from build123d import *

# Parameters (mm, degrees)
SM_BASE_FLANGE_2_DEPTH = 20
HOLE_WIZARD_M3_1_D     = 3.2
SKETCH_24_R            = 3.6
CUT_EXTRUDE_2_DEPTH    = 67.332495807
HOLE_WIZARD_M4_1_D     = 4.3
HOLE_WIZARD_M2_5_1_D   = 2.7


# Sheet-metal steps are written as plain solids
with BuildPart() as part:
    # 草圖16 → 基材-凸緣2 (new, symmetric)
    with BuildSketch(Plane.XY):
        with BuildLine():
            Line((36, 0), (1, 0))
            ThreePointArc((1, 0), (0.292893219, 0.292893219), (0, 1))
            Line((0, 1), (0, 48))
            Line((0, 48), (-4, 48))
            Line((-4, 48), (-4, 1))
            ThreePointArc((-4, 1), (-2.535533906, -2.535533906), (1, -4))
            Line((1, -4), (36, -4))
            Line((36, -4), (36, 0))
        make_face()
    extrude(amount=SM_BASE_FLANGE_2_DEPTH, both=True)

    # M3 餘隙孔1 (through all)
    with Locations(Plane(origin=(0, 0, 0), x_dir=(-1, 0, 0), z_dir=(0, 1, 0))):
        with Locations((-27, 17.5), (-11, 2.5), (-11, 17.5), (-27, 2.5)):
            Hole(HOLE_WIZARD_M3_1_D / 2)

    # 草圖24 → 除料-伸長2 (cut, through all)
    with BuildSketch(Plane.XZ.offset(4)):
        with Locations(Location((19, -10, 0), (0, 0, 270))):
            Circle(SKETCH_24_R)
    extrude(amount=-CUT_EXTRUDE_2_DEPTH, mode=Mode.SUBTRACT)

    # M4 餘隙孔1 (through all)
    with Locations(Plane(origin=(0, 0, 0), x_dir=(0, 0, 1), z_dir=(1, 0, 0))):
        with Locations((0, -44), (15, -44), (15, -24), (0, -24)):
            Hole(HOLE_WIZARD_M4_1_D / 2)

    # M2.5 餘隙孔1 (through all)
    with Locations(Plane(origin=(0, -4, 0), x_dir=(-1, 0, 0), z_dir=(0, -1, 0))):
        with Locations((-11.5, 10), (-26.5, 10)):
            Hole(HOLE_WIZARD_M2_5_1_D / 2)


solid = part.part
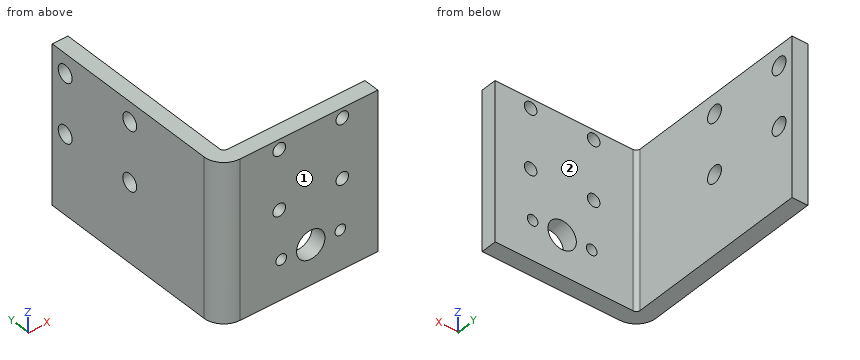
Build history of the part. All positions in model axes, mm. Face numbers are marked on the shaded views. A direction names the side the tool comes from. Round coordinates to 2 decimals unless told otherwise and drop trailing zeros. Loops run counter-clockwise (first coordinate to the right, second up) from the corner with the lowest first, then second, coordinate; pieces in that order, holes last. Notation, with made-up numbers: (74, -10.75) -> (121, -10.75) arc R17 ccw to (121, 13.25) -> close; hole circle Ø7 at (0, 57). An arc over 180 degrees is marked (long way). Answer in a Markdown table with one row per item.
Item 1: Which spindle directions (+Z, -Z, +X, -X, +Y, -Y) get a long thin tool onto all of the face, cutting with end or side? Do the marked faces 1 and 2. Say none if no direction does.
Answers below:
| item | result |
|---|---|
| face 1 | +Z, -Z, +X, -X, -Y |
| face 2 | +Z, -Z, +X, +Y |
Item 2: Saw through at B-B (x = 27). Write the cut outline in (y, z), and give its area (3 significant figures).
Answers below:
| item | result |
|---|---|
| outline | (-4, -20) -> (0, -20) -> (0, -11.25) -> (-4, -11.25) -> close; (-4, -8.75) -> (0, -8.75) -> (0, 0.9) -> (-4, 0.9) -> close; (-4, 4.1) -> (0, 4.1) -> (0, 15.9) -> (-4, 15.9) -> close; (-4, 19.1) -> (0, 19.1) -> (0, 20) -> (-4, 20) -> close |
| area | 124 mm² |
Item 3: Saw through at D-D (z = -10). Write the cut outline in (x, y), and give its area (3 significant figures).
Answers below:
| item | result |
|---|---|
| outline | (-4, 1) arc R5 ccw to (1, -4) -> (10.15, -4) -> (10.15, 0) -> (1, 0) arc R1 cw to (0, 1) -> (0, 48) -> (-4, 48) -> close; (12.85, -4) -> (15.4, -4) -> (15.4, 0) -> (12.85, 0) -> close; (22.6, -4) -> (25.15, -4) -> (25.15, 0) -> (22.6, 0) -> close; (27.85, -4) -> (36, -4) -> (36, 0) -> (27.85, 0) -> close |
| area | 296 mm² |
Item 4: Drill centre lines: L1, parallel to Z at x = -2.55, y = 44; L2, parallel to X at y = -3.1, z = -10; L3, parallel to Y at x = -1, z = 0. Where is each one in solid material? Low to high. Write a range as [from, to].
Answers below:
| item | result |
|---|---|
| L1 | z = [-20, -2.15], [2.15, 12.85], [17.15, 20] |
| L2 | x = [-1.86, 10.15], [12.85, 15.4], [22.6, 25.15], [27.85, 36] |
| L3 | y = [-3.58, 21.85], [26.15, 41.85], [46.15, 48] |
Item 5: Pin check, flat tips, straight feed: pin 1 (5.5 mm diameter, centred on y = 44, z = 15, fed in from +X); pin 2 (2 mm diameter, centred on x = 26.5, z = -10, fed in from -Y); pin 3 (10 mm diameter, centred on x = 12.5, z = -11, fed in from +Y). Stop position of each tip, or through.
Answers below:
| item | result |
|---|---|
| pin 1 | stops at x = 0 |
| pin 2 | passes through |
| pin 3 | stops at y = 0 |
Item 6: Saw through at A-A (z = 0). Write the cut outline in (x, y), and give its area (3 significant figures).
Answers below:
| item | result |
|---|---|
| outline | (-4, 1) arc R5 ccw to (1, -4) -> (36, -4) -> (36, 0) -> (1, 0) arc R1 cw to (0, 1) -> (0, 21.85) -> (-4, 21.85) -> close; (-4, 26.15) -> (0, 26.15) -> (0, 41.85) -> (-4, 41.85) -> close; (-4, 46.15) -> (0, 46.15) -> (0, 48) -> (-4, 48) -> close |
| area | 312 mm² |
Item 7: Saw through at C-C (y = 24). Write the cut outline in (x, z), and give its area (3 significant figures).
Answers below:
| item | result |
|---|---|
| outline | (-4, -20) -> (0, -20) -> (0, -2.15) -> (-4, -2.15) -> close; (-4, 2.15) -> (0, 2.15) -> (0, 12.85) -> (-4, 12.85) -> close; (-4, 17.15) -> (0, 17.15) -> (0, 20) -> (-4, 20) -> close |
| area | 126 mm² |
